Can you work these out from the model? Positions are in its coordinate system, mm. Face numbers are marked on the shaded views. A direction names the side the tool comes from. Give positions to 0.01 mm unless a question says otherwise; leave off trailing zeros. Write each loop counter-clockwise with the first axis right and the second up, starting at its lowest first coordinate (ties: lowest second). Pieces come first, ordered by that corner, then holes. Notation, with made-up numbers: (-33, -5.5) - (11, -5.5) arc R20 cw to (11, 8.5) - close; hole circle Ø2 at (-10, 23.5). An arc over 180 degrees is marked (long way). Return JSON: item names as keys, results as strings. Group by question number.
from build123d import *

# Parameters (mm, degrees)
SKETCH1_R           = 3.5
SKETCH1_R_2         = 2.5
BOSS_EXTRUDE1_DEPTH = 4
BOSS_EXTRUDE2_START = -2
SKETCH2_R           = 3.5
SKETCH2_R_2         = 1
BOSS_EXTRUDE2_DEPTH = 1.5
BOSS_EXTRUDE3_START = -1
BOSS_EXTRUDE3_DEPTH = 1
CUT_EXTRUDE1_REACH  = 18.86
SKETCH4_R           = 0.5


with BuildPart() as part:
    # Sketch1 → Boss-Extrude1 (new body)
    with BuildSketch(Plane(origin=(0, 0, 0), x_dir=(1, 0, 0), z_dir=(0, 1, 0))):
        with Locations(Location((0, 0, 0), (0, 0, 270))):
            Circle(SKETCH1_R)
        with Locations(Location((0, 0, 0), (0, 0, 270))):
            Circle(SKETCH1_R_2, mode=Mode.SUBTRACT)
    extrude(amount=BOSS_EXTRUDE1_DEPTH)

    # Sketch2 → Boss-Extrude2 (add)
    with BuildSketch(Plane(origin=(0, 4, 0), x_dir=(1, 0, 0), z_dir=(0, 1, 0)).offset(BOSS_EXTRUDE2_START)):
        with Locations(Location((0, 0, 0), (0, 0, 270))):
            Circle(SKETCH2_R)
        with Locations(Location((0, 0, 0), (0, 0, 270))):
            Circle(SKETCH2_R_2, mode=Mode.SUBTRACT)
    extrude(amount=BOSS_EXTRUDE2_DEPTH)

    # Sketch3 → Boss-Extrude3 (add)
    with BuildSketch(Plane(origin=(0, 4, 0), x_dir=(1, 0, 0), z_dir=(0, 1, 0)).offset(BOSS_EXTRUDE3_START)):
        with BuildLine():
            ThreePointArc((-2.449489743, -2.5), (-3.5, 0), (-2.449489743, 2.5))
            Line((-2.449489743, 2.5), (-14.086174253, 1.998142637))
            ThreePointArc((-14.086174253, 1.998142637), (-16, 0), (-14.086174253, -1.998142637))
            Line((-14.086174253, -1.998142637), (-2.449489743, -2.5))
        make_face()
        with BuildLine():
            Line((2.449489743, -2.5), (14.086174253, -1.998142637))
            ThreePointArc((14.086174253, -1.998142637), (16, 0), (14.086174253, 1.998142637))
            Line((14.086174253, 1.998142637), (2.449489743, 2.5))
            ThreePointArc((2.449489743, 2.5), (3.5, 0), (2.449489743, -2.5))
        make_face()
    extrude(amount=BOSS_EXTRUDE3_DEPTH)

    # Sketch4 → Cut-Extrude1 (cut, up to next)
    with BuildSketch(Plane(origin=(0, 4, 0), x_dir=(1, 0, 0), z_dir=(0, 1, 0)), mode=Mode.PRIVATE) as cut_extrude1_sk1:
        with Locations(Location((4, 0, 0), (0, 0, 270))):
            Circle(SKETCH4_R)
    cut_extrude1_tool1 = extrude(cut_extrude1_sk1.sketch, amount=-CUT_EXTRUDE1_REACH, mode=Mode.PRIVATE) & part.part
    # Sketch4 → Cut-Extrude1 (cut, up to next)
    with BuildSketch(Plane(origin=(0, 4, 0), x_dir=(1, 0, 0), z_dir=(0, 1, 0)), mode=Mode.PRIVATE) as cut_extrude1_sk2:
        with Locations(Location((6, 0, 0), (0, 0, 270))):
            Circle(SKETCH4_R)
    cut_extrude1_tool2 = extrude(cut_extrude1_sk2.sketch, amount=-CUT_EXTRUDE1_REACH, mode=Mode.PRIVATE) & part.part
    # Sketch4 → Cut-Extrude1 (cut, up to next)
    with BuildSketch(Plane(origin=(0, 4, 0), x_dir=(1, 0, 0), z_dir=(0, 1, 0)), mode=Mode.PRIVATE) as cut_extrude1_sk3:
        with Locations(Location((8, 0, 0), (0, 0, 270))):
            Circle(SKETCH4_R)
    cut_extrude1_tool3 = extrude(cut_extrude1_sk3.sketch, amount=-CUT_EXTRUDE1_REACH, mode=Mode.PRIVATE) & part.part
    # Sketch4 → Cut-Extrude1 (cut, up to next)
    with BuildSketch(Plane(origin=(0, 4, 0), x_dir=(1, 0, 0), z_dir=(0, 1, 0)), mode=Mode.PRIVATE) as cut_extrude1_sk4:
        with Locations(Location((10, 0, 0), (0, 0, 270))):
            Circle(SKETCH4_R)
    cut_extrude1_tool4 = extrude(cut_extrude1_sk4.sketch, amount=-CUT_EXTRUDE1_REACH, mode=Mode.PRIVATE) & part.part
    # Sketch4 → Cut-Extrude1 (cut, up to next)
    with BuildSketch(Plane(origin=(0, 4, 0), x_dir=(1, 0, 0), z_dir=(0, 1, 0)), mode=Mode.PRIVATE) as cut_extrude1_sk5:
        with Locations(Location((12, 0, 0), (0, 0, 270))):
            Circle(SKETCH4_R)
    cut_extrude1_tool5 = extrude(cut_extrude1_sk5.sketch, amount=-CUT_EXTRUDE1_REACH, mode=Mode.PRIVATE) & part.part
    # Sketch4 → Cut-Extrude1 (cut, up to next)
    with BuildSketch(Plane(origin=(0, 4, 0), x_dir=(1, 0, 0), z_dir=(0, 1, 0)), mode=Mode.PRIVATE) as cut_extrude1_sk6:
        with Locations(Location((14, 0, 0), (0, 0, 270))):
            Circle(SKETCH4_R)
    cut_extrude1_tool6 = extrude(cut_extrude1_sk6.sketch, amount=-CUT_EXTRUDE1_REACH, mode=Mode.PRIVATE) & part.part
    # Sketch4 → Cut-Extrude1 (cut, up to next)
    with BuildSketch(Plane(origin=(0, 4, 0), x_dir=(1, 0, 0), z_dir=(0, 1, 0)), mode=Mode.PRIVATE) as cut_extrude1_sk7:
        with Locations(Location((-14, 0, 0), (0, 0, 270))):
            Circle(SKETCH4_R)
    cut_extrude1_tool7 = extrude(cut_extrude1_sk7.sketch, amount=-CUT_EXTRUDE1_REACH, mode=Mode.PRIVATE) & part.part
    # Sketch4 → Cut-Extrude1 (cut, up to next)
    with BuildSketch(Plane(origin=(0, 4, 0), x_dir=(1, 0, 0), z_dir=(0, 1, 0)), mode=Mode.PRIVATE) as cut_extrude1_sk8:
        with Locations(Location((-12, 0, 0), (0, 0, 270))):
            Circle(SKETCH4_R)
    cut_extrude1_tool8 = extrude(cut_extrude1_sk8.sketch, amount=-CUT_EXTRUDE1_REACH, mode=Mode.PRIVATE) & part.part
    # Sketch4 → Cut-Extrude1 (cut, up to next)
    with BuildSketch(Plane(origin=(0, 4, 0), x_dir=(1, 0, 0), z_dir=(0, 1, 0)), mode=Mode.PRIVATE) as cut_extrude1_sk9:
        with Locations(Location((-10, 0, 0), (0, 0, 270))):
            Circle(SKETCH4_R)
    cut_extrude1_tool9 = extrude(cut_extrude1_sk9.sketch, amount=-CUT_EXTRUDE1_REACH, mode=Mode.PRIVATE) & part.part
    # Sketch4 → Cut-Extrude1 (cut, up to next)
    with BuildSketch(Plane(origin=(0, 4, 0), x_dir=(1, 0, 0), z_dir=(0, 1, 0)), mode=Mode.PRIVATE) as cut_extrude1_sk10:
        with Locations(Location((-8, 0, 0), (0, 0, 270))):
            Circle(SKETCH4_R)
    cut_extrude1_tool10 = extrude(cut_extrude1_sk10.sketch, amount=-CUT_EXTRUDE1_REACH, mode=Mode.PRIVATE) & part.part
    # Sketch4 → Cut-Extrude1 (cut, up to next)
    with BuildSketch(Plane(origin=(0, 4, 0), x_dir=(1, 0, 0), z_dir=(0, 1, 0)), mode=Mode.PRIVATE) as cut_extrude1_sk11:
        with Locations(Location((-6, 0, 0), (0, 0, 270))):
            Circle(SKETCH4_R)
    cut_extrude1_tool11 = extrude(cut_extrude1_sk11.sketch, amount=-CUT_EXTRUDE1_REACH, mode=Mode.PRIVATE) & part.part
    # Sketch4 → Cut-Extrude1 (cut, up to next)
    with BuildSketch(Plane(origin=(0, 4, 0), x_dir=(1, 0, 0), z_dir=(0, 1, 0)), mode=Mode.PRIVATE) as cut_extrude1_sk12:
        with Locations(Location((-4, 0, 0), (0, 0, 359.998928085))):
            Circle(SKETCH4_R)
    cut_extrude1_tool12 = extrude(cut_extrude1_sk12.sketch, amount=-CUT_EXTRUDE1_REACH, mode=Mode.PRIVATE) & part.part
    add(cut_extrude1_tool1.solids().sort_by_distance((4, 4, 0))[0], mode=Mode.SUBTRACT)
    add(cut_extrude1_tool2.solids().sort_by_distance((6, 4, 0))[0], mode=Mode.SUBTRACT)
    add(cut_extrude1_tool3.solids().sort_by_distance((8, 4, 0))[0], mode=Mode.SUBTRACT)
    add(cut_extrude1_tool4.solids().sort_by_distance((10, 4, 0))[0], mode=Mode.SUBTRACT)
    add(cut_extrude1_tool5.solids().sort_by_distance((12, 4, 0))[0], mode=Mode.SUBTRACT)
    add(cut_extrude1_tool6.solids().sort_by_distance((14, 4, 0))[0], mode=Mode.SUBTRACT)
    add(cut_extrude1_tool7.solids().sort_by_distance((-14, 4, 0))[0], mode=Mode.SUBTRACT)
    add(cut_extrude1_tool8.solids().sort_by_distance((-12, 4, 0))[0], mode=Mode.SUBTRACT)
    add(cut_extrude1_tool9.solids().sort_by_distance((-10, 4, 0))[0], mode=Mode.SUBTRACT)
    add(cut_extrude1_tool10.solids().sort_by_distance((-8, 4, 0))[0], mode=Mode.SUBTRACT)
    add(cut_extrude1_tool11.solids().sort_by_distance((-6, 4, 0))[0], mode=Mode.SUBTRACT)
    add(cut_extrude1_tool12.solids().sort_by_distance((-4, 4, 0))[0], mode=Mode.SUBTRACT)


solid = part.part
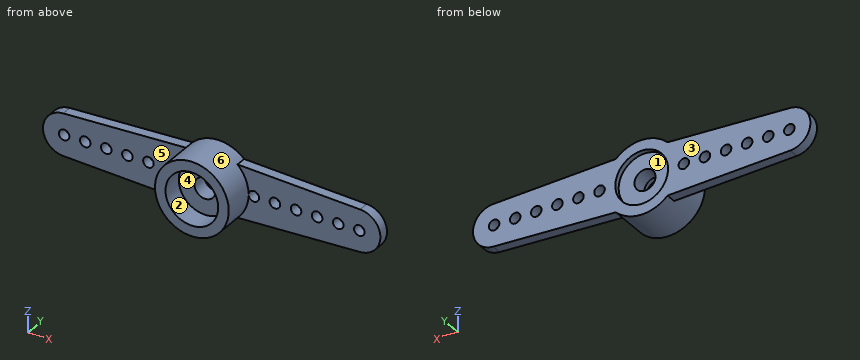
1) Imagine slicing it at B-B, the plane y = 1.7. Write out the boundary of the cut face in (x, z), and give its area (3 significant figures).
2) On a 3-axis mill with a long thin cutter (end or side, diameter ignored), from which of +Z, -Z, +X, -X, +Y, -Y can I reach the whole of each face in a straight line? I mean the marked faces 1, 2 and 3. Say none if no direction works.
3) Will these pins go through, and if not, where does the flat tip stop? pin 1 Ø2 at (x, y) = (3.5, 3) entering from +Z; pin 2 Ø2.5 at (x, z) = (-0.5, 0) entering from -Y; pin 3 Ø4 at (x, z) = (10, 0) entering from -Y.
4) Imagine slicing it at A-A, the plane x = 12. Write out the boundary of the cut face in (y, z), and give its area (3 significant figures).
5) Imagine slicing it at D-D, the plane x = 2. Write out the boundary of the cut face in (y, z), and give its area (3 significant figures).
6) Imagine slicing it at C-C, the plane x = 8. Write out the boundary of the cut face in (y, z), and give its area (3 significant figures).
7) I need wall thicknesses on line 1 along Z through (x, y) = (0, 3.85); line 2 along Y through (x, z) = (11, 0.5); line 3 along Y through (x, z) = (-2, -0.75). Which ranges of each line are inside material? Lowest first, please.
8) We'd pull the mould along X, two halves only. Please class the marked faces 4, 5 and 6: pulls with the +X half, pulls with the -X half, needs draft (parallel to the pull), parting line crosses it, or undercut.
Resolved:
{
 "1": {"outline": "circle Ø7 at (0, 0); hole circle Ø5 at (0, 0)", "area": "18.8 mm^2"},
 "2": {"face 1": "+Y", "face 2": "-Y", "face 3": "+Z, -Z, +X, -X, +Y"},
 "3": {"pin 1": "z = 2.5", "pin 2": "y = 2", "pin 3": "y = 3"},
 "4": {"outline": "(3, -2.09) - (4, -2.09) - (4, -0.5) - (3, -0.5) - close; (3, 0.5) - (4, 0.5) - (4, 2.09) - (3, 2.09) - close", "area": "3.18 mm^2"},
 "5": {"outline": "(0, -2.87) - (4, -2.87) - (4, -1.5) - (3.5, -1.5) - (3.5, 1.5) - (4, 1.5) - (4, 2.87) - (0, 2.87) - (0, 1.5) - (2, 1.5) - (2, -1.5) - (0, -1.5) - close", "area": "15.5 mm^2"},
 "6": {"outline": "(3, -2.26) - (4, -2.26) - (4, -0.5) - (3, -0.5) - close; (3, 0.5) - (4, 0.5) - (4, 2.26) - (3, 2.26) - close", "area": "3.52 mm^2"},
 "7": {"line 1": "-3.5 to -2.5, 2.5 to 3.5", "line 2": "3 to 4", "line 3": "2 to 3.5"},
 "8": {"face 4": "undercut", "face 5": "needs draft", "face 6": "parting line crosses it"}
}
